CAD build for the part. Positions are in the model's coordinates, mm. Face numbers are marked on the shaded views. Round coordinates to 2 decimals unless told otherwise and drop trailing zeros. Order: outer loops, then holes, each group sorted by start corner. A loop starts at its lowest first (then second) coordinate and runs counter-clockwise, first axis right, second up.
```python
from build123d import *

# Parameters (mm, degrees)
SKETCH1_W           = 52
SKETCH1_H           = 15
BOSS_EXTRUDE1_DEPTH = 6.35
SKETCH3_R           = 2
CUT_EXTRUDE2_DEPTH  = 28.795188433
SKETCH2_W           = 26
SKETCH2_H           = 15
CUT_EXTRUDE1_DEPTH  = 28.795188433


with BuildPart() as part:
    # Sketch1 → Boss-Extrude1 (new body)
    with BuildSketch(Plane(origin=(0, 0, 0), x_dir=(1, 0, 0), z_dir=(0, 1, 0))):
        Rectangle(SKETCH1_W, SKETCH1_H)
    extrude(amount=BOSS_EXTRUDE1_DEPTH)

    # Sketch3 → Cut-Extrude2 (cut, through all)
    with BuildSketch(Plane(origin=(0, 6.35, 0), x_dir=(1, 0, 0), z_dir=(0, 1, 0))):
        with Locations(Location((-13, 0, 0), (0, 0, 270))):
            Circle(SKETCH3_R)
        with Locations(Location((13, 0, 0), (0, 0, 270))):
            Circle(SKETCH3_R)
    extrude(amount=-CUT_EXTRUDE2_DEPTH, mode=Mode.SUBTRACT)

    # Sketch2 → Cut-Extrude1 (cut, through all)
    with BuildSketch(Plane(origin=(0, 6.35, 0), x_dir=(1, 0, 0), z_dir=(0, 1, 0))):
        with Locations((13, 0)):
            Rectangle(SKETCH2_W, SKETCH2_H)
    extrude(amount=-CUT_EXTRUDE1_DEPTH, mode=Mode.SUBTRACT)


solid = part.part
```
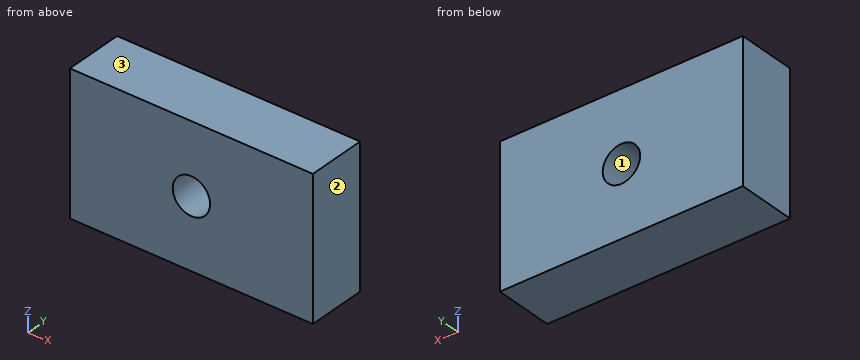
1. Cut at A-A, the plane x = -13. Write the cut outline in (y, z).
2. Mould opens along X. For the marked faces 1, 2 and 3 say: released by +X, released by -X, zero draft, split by the parting line, or undercut.
3. Drill centre lines: line 1 (X direction, y = 1.5, z = 0); line 2 (Z direction, x = -13.25, y = 2.25); line 3 (X direction, y = 1.25, z = 0.5). Where is each one in solid material? Low to high.
4. Cut at C-C, the plane y = 4.75. Write the cut outline in (x, z).
5. Cut at B-B, the plane z = 0. Write the cut outline in (x, y).
Outcome:
1. outline: (0, -7.5) - (6.35, -7.5) - (6.35, -2) - (0, -2) - close; (0, 2) - (6.35, 2) - (6.35, 7.5) - (0, 7.5) - close
2. face 1: undercut
2. face 2: released by +X
2. face 3: zero draft
3. line 1: x = -26 to -15, -11 to 0
3. line 2: z = -7.5 to -1.98, 1.98 to 7.5
3. line 3: x = -26 to -14.94, -11.06 to 0
4. outline: (-26, -7.5) - (0, -7.5) - (0, 7.5) - (-26, 7.5) - close; hole circle Ø4 at (-13, 0)
5. outline: (-26, 0) - (-15, 0) - (-15, 6.35) - (-26, 6.35) - close; (-11, 0) - (0, 0) - (0, 6.35) - (-11, 6.35) - close
